Geometry: final body of the model. Coordinates: model frame, mm. Face numbers are marked on the shaded views. Coordinates: 2 decimals unless noted, no trailing zeros. Order: outer loops, then holes, each group sorted by start corner. A loop starts at its lowest first (then second) coordinate and runs counter-clockwise, first axis right, second up. Notation, with made-up numbers: (42, -29.75) -> (91, -29.75) arc R28 ccw to (91, 6.25) -> close; hole circle Ø7 at (26, -3.75). An arc over 180 degrees is marked (long way). Answer in a Markdown table with one row per item. Add a question column.
1) Ray query, line 1 (X direction, y = 4, z = -1.5); line 2 (Z direction, x = -41, y = -94). Return the intervals inside material, ascending. Write a range as from..to.
2) Pull-direction query (X, two-part tool) for the marked faces 1 and 2; classes: +X half, -X half, draft (parallel to the pull), parting line (faces both ways), or undercut.
3) Section query A-A on z = -3.25. Return the cut outline in (x, y).
4) Contact query for flat-ended pins moving along their axis: P1, Ø4, axis at x = 82, z = -2.5, coming from the +Y side; P2, Ø4, axis at x = 77.84, y = -61.62, coming from the -Z side. Output: stop coordinate, or through.
5) Section query C-C on x = -12. Return the cut outline in (y, z).
6) Section query D-D on y = -23.5. Return the cut outline in (x, z).
7) Section query B-B on y = -106. Return the cut outline in (x, z), then the cut area to 3 significant figures.
```python
from build123d import *

# Parameters (mm, degrees)
SKETCH_1_W      = 138
SKETCH_1_H      = 141
SKETCH_1_R      = 1.6
EXTRUDE_1_DEPTH = 3
SKETCH_2_W      = 5
SKETCH_2_H      = 20
EXTRUDE_2_DEPTH = 6


with BuildPart() as part:
    # 草图1 → 凸台-拉伸1 (new body)
    with BuildSketch(Plane.XY):
        with Locations((14.838842975, -46.124397743)):
            Rectangle(SKETCH_1_W, SKETCH_1_H)
        with Locations((-48.161157025, 18.375602257)):
            Circle(SKETCH_1_R, mode=Mode.SUBTRACT)
        with Locations((77.838842975, 18.375602257)):
            Circle(SKETCH_1_R, mode=Mode.SUBTRACT)
        with Locations((-48.161157025, -61.624397743)):
            Circle(SKETCH_1_R, mode=Mode.SUBTRACT)
        with Locations((77.838842975, -61.624397743)):
            Circle(SKETCH_1_R, mode=Mode.SUBTRACT)
    extrude(amount=EXTRUDE_1_DEPTH)

    # 草图2 → 凸台-拉伸2 (add)
    with BuildSketch(Plane(origin=(0, 0, 0), x_dir=(-1, 0, 0), z_dir=(0, 0, -1))):
        with Locations((-81.338842975, -106.624397743)):
            Rectangle(SKETCH_2_W, SKETCH_2_H)
        with Locations((-81.338842975, -0.534764205)):
            Rectangle(SKETCH_2_W, SKETCH_2_H)
        with Locations((51.661157025, -106.624397743)):
            Rectangle(SKETCH_2_W, SKETCH_2_H)
        with Locations((51.661157025, -0.534764205)):
            Rectangle(SKETCH_2_W, SKETCH_2_H)
    extrude(amount=EXTRUDE_2_DEPTH)


solid = part.part
```
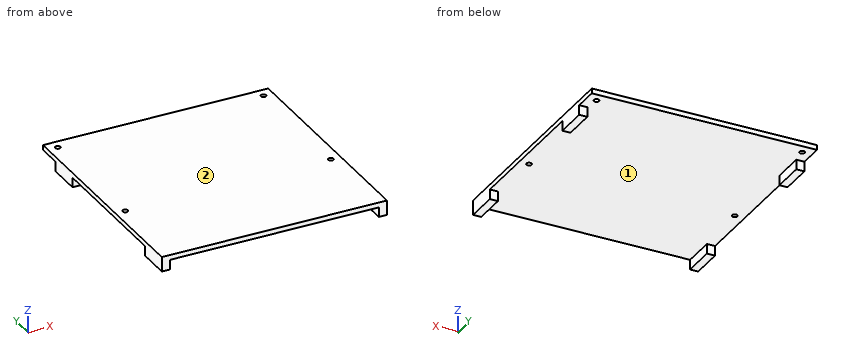
Result:
| question | item | result |
|---|---|---|
| 1 | line 1 | -54.16..-49.16, 78.84..83.84 |
| 1 | line 2 | 0..3 |
| 2 | face 1 | undercut |
| 2 | face 2 | draft |
| 3 | outline | (-54.16, -116.62) -> (-49.16, -116.62) -> (-49.16, -96.62) -> (-54.16, -96.62) -> close; (-54.16, -10.53) -> (-49.16, -10.53) -> (-49.16, 9.47) -> (-54.16, 9.47) -> close; (78.84, -116.62) -> (83.84, -116.62) -> (83.84, -96.62) -> (78.84, -96.62) -> close; (78.84, -10.53) -> (83.84, -10.53) -> (83.84, 9.47) -> (78.84, 9.47) -> close |
| 4 | P1 | y = 9.47 |
| 4 | P2 | z = 0 |
| 5 | outline | (-116.62, 0) -> (24.38, 0) -> (24.38, 3) -> (-116.62, 3) -> close |
| 6 | outline | (-54.16, 0) -> (83.84, 0) -> (83.84, 3) -> (-54.16, 3) -> close |
| 7 | outline | (-54.16, -6) -> (-49.16, -6) -> (-49.16, 0) -> (78.84, 0) -> (78.84, -6) -> (83.84, -6) -> (83.84, 3) -> (-54.16, 3) -> close |
| 7 | area | 474 mm2 |
